Here's the drawing with two shaded views (mm, measured from the low corner). I have some questions. A direction names the side the tool comes from. Round coordinates to 2 decimals unless told otherwise and drop trailing zeros. Order: outer loops, then holes, each group sorted by start corner. A loop starts at its lowest first (then second) coordinate and runs counter-clockwise, first axis right, second up. Notation, with made-up numbers: (63, 85.5) -> (118, 85.5) arc R23 cw to (118, 121.5) -> close; hole circle Ø11 at (-24, 24.25). An arc over 180 degrees is marked (long way). Put each result on its own line as item: value. Start each with the question number.
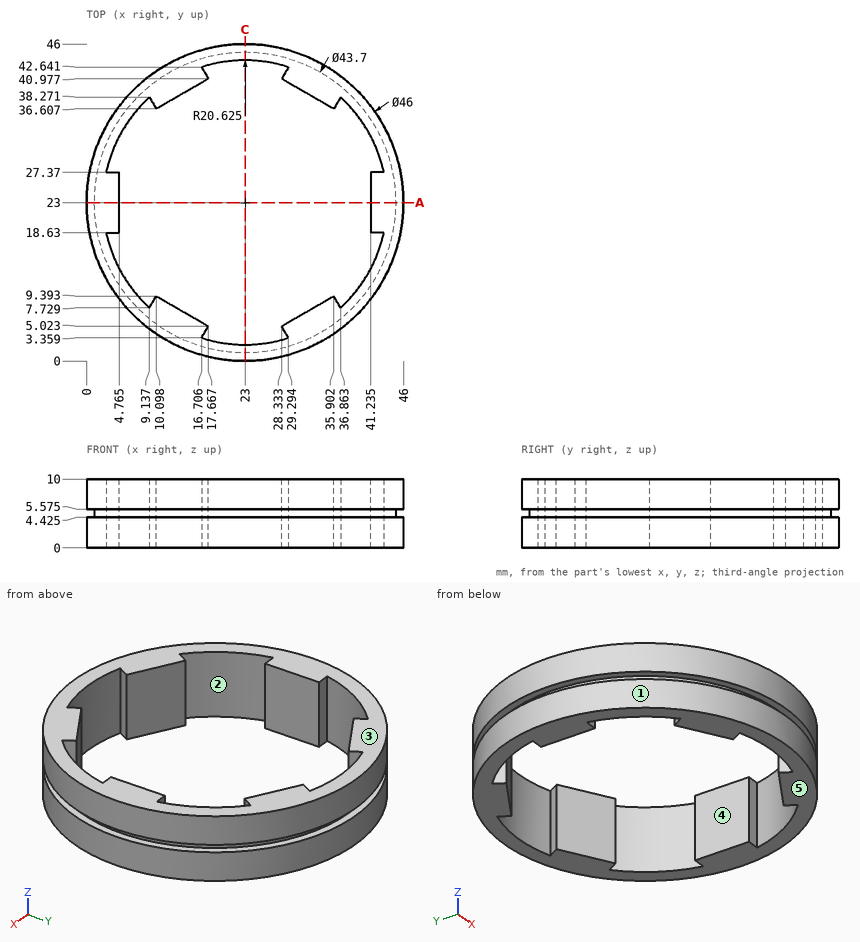
1. For pin 1 Ø4 at (y, z) = (34, 8.5) entering from +X; pin 2 Ø1.5 at (x, z) = (4, 6.5) entering from +Y; pin 3 Ø0.6 at (x, z) = (42.5, 5.5) entering from +Y, each with a flat end and sliding along its axis, tell me the tip position at first contact or that it passes through.
2. Thinking about a two-plate mould opening in Y: for the marked faces 1, 2 and 3, which applies, +Y half, -Y half, draft (parallel to the pull), parting line (faces both ways), or undercut?
3. I need wall thicknesses on L1, parallel to Y at x = 4, z = 4 (1 decimal); L2, parallel to Y at x = 23, z = 7 (3 decimals); L3, parallel to Y at x = 29, z = 9.25 (1 decimal). Which ranges of each line are inside material? Lowest first, please.
4. If we section it at A-A, the plane y = 23: Please give me the cut outline in (x, z) (3 decimals).
5. Which directions (+Z, -Z, +X, -X, +Y, -Y) give clear straight access to the entire face, cutting with the end or side of a thin tool? Please do the marked faces 4 and 5.
6. If we section it at C-C, the plane x = 23: Please give me the cut outline in (y, z) (3 decimals).
Results below:
1. pin 1: x = 44.17
1. pin 2: y = 37
1. pin 3: y = 35.65
2. face 1: parting line
2. face 2: undercut
2. face 3: draft
3. L1: 10 to 15, 18.6 to 27.4, 31 to 36
3. L2: 0 to 2.375, 43.625 to 46
3. L3: 0.8 to 3.3, 3.9 to 5.4, 40.6 to 42.1, 42.7 to 45.2
4. outline: (0, 0) -> (4.765, 0) -> (4.765, 10) -> (0, 10) -> (0, 5.575) -> (1.15, 5.575) -> (1.15, 4.425) -> (0, 4.425) -> close; (41.235, 0) -> (46, 0) -> (46, 4.425) -> (44.85, 4.425) -> (44.85, 5.575) -> (46, 5.575) -> (46, 10) -> (41.235, 10) -> close
5. face 4: +Z, -Z
5. face 5: -Z, +X, -X, +Y, -Y
6. outline: (0, 0) -> (2.375, 0) -> (2.375, 10) -> (0, 10) -> (0, 5.575) -> (1.15, 5.575) -> (1.15, 4.425) -> (0, 4.425) -> close; (43.625, 0) -> (46, 0) -> (46, 4.425) -> (44.85, 4.425) -> (44.85, 5.575) -> (46, 5.575) -> (46, 10) -> (43.625, 10) -> close
